from build123d import *

# Parameters (mm, degrees)
SALIENTE_EXTRUIR1_DEPTH = 10
CROQUIS2_R              = 2
CORTAR_EXTRUIR1_DEPTH   = 10
CROQUIS3_R              = 2
CORTAR_EXTRUIR2_DEPTH   = 10


with BuildPart() as part:
    # Croquis1 → Saliente-Extruir1 (new body)
    with BuildSketch(Plane(origin=(0, 0, 0), x_dir=(0, 0, -1), z_dir=(1, 0, 0))):
        Polygon((0, 0), (37.42423058, 37.42423058), (50, 0), align=None)
    extrude(amount=SALIENTE_EXTRUIR1_DEPTH)

    # Croquis2 → Cortar-Extruir1 (cut)
    with BuildSketch(Plane.XZ):
        with Locations(Location((5, -34.477712546, 0), (0, 0, 270))):
            Circle(CROQUIS2_R)
    extrude(amount=-CORTAR_EXTRUIR1_DEPTH, mode=Mode.SUBTRACT)

    # Croquis3 → Cortar-Extruir2 (cut)
    with BuildSketch(Plane(origin=(0, 0, 0), x_dir=(1, 0, 0), z_dir=(0, 0.7071067811865512, 0.7071067811865439))):
        with Locations(Location((5, 42.766502378, 0), (0, 0, 270))):
            Circle(CROQUIS3_R)
    extrude(amount=-CORTAR_EXTRUIR2_DEPTH, mode=Mode.SUBTRACT)


solid = part.part
The listing builds one solid part. Answer for the finished solid, in the listing's coordinates (mm). A direction names the side the tool comes from. Give positions to 0.01 mm unless a question says otherwise; leave off trailing zeros. Loops run counter-clockwise (first coordinate to the right, second up) from the corner with the lowest first, then second, coordinate; pieces in that order, holes last.
Item 1: Each of these flat-tipped pins is pushed along its axis until it touches: pin 1 Ø6 at (x, y) = (6.5, 12.5) entering from +Z; pin 2 Ø2 at (x, y) = (6.5, 11.5) entering from -Z; pin 3 Ø3 at (x, z) = (5, -34.48) entering from +Y. Where does it stop, or does it pass through?
Derived:
pin 1: stops at z = -9.5
pin 2: stops at z = -46.47
pin 3: stops at y = 35.98
Item 2: A cutting plane is placed at D-D (x = 1). Give the vertices of the cut face in (y, z).
Derived:
outline: (0, -50) - (37.42, -37.42) - (0, 0) - close
Item 3: A tool of negligible diameter and unlimited length cuts with its end or side. For faces 1 (the flat face through (0, 11, -31)), 2 (the flat face through (5.03, 23.19, -37.33)), 3 (the flat face through (5, 10, -34)), from which of +Z, -Z, +X, -X, +Y, -Y can it reach the whole face along a straight path? Write none if from no direction.
Derived:
face 1: +Z, -Z, -X, +Y, -Y
face 2: none
face 3: -Y
Item 4: Find the intervals of material crossed by line 1 along Z through (x, y) = (3.5, 28); line 2 along Y through (x, z) = (8.5, -10); line 3 along Z through (x, y) = (3, 16.5), in increasing order.
Derived:
line 1: z = -40.59 to -34.35, -30.61 to -28
line 2: y = 0 to 10
line 3: z = -44.46 to -16.5
Item 5: A cutting plane is placed at B-B (z = -21). Give the vertices of the cut face in (x, y), then the cut area to 3 significant figures.
Derived:
outline: (0, 0) - (10, 0) - (10, 21) - (0, 21) - close
area: 210 mm2
Item 6: Determine the mould class of faces 4 (the cylindrical face through (5.601, 4.93, -36.385)), 5 (the flat face through (5, 0, -25)), 6 (the cylindrical face through (6.35, 27.8, -34.77)) for opening direction Y: +Y half, -Y half, draft (parallel to the pull), parting line (faces both ways), or undercut.
Derived:
face 4: draft
face 5: -Y half
face 6: undercut
Item 7: A cutting plane is placed at A-A (x = 5). Give the vertices of the cut face in (y, z).
Derived:
outline: (0, -50) - (37.42, -37.42) - (31.65, -31.65) - (24.58, -38.73) - (21.76, -35.9) - (28.83, -28.83) - (0, 0) - (0, -32.48) - (10, -32.48) - (10, -36.48) - (0, -36.48) - close
Item 8: A cutting plane is placed at C-C (y = 14.5). Give the vertices of the cut face in (x, z), then the cut area to 3 significant figures.
Derived:
outline: (0, -45.13) - (10, -45.13) - (10, -14.5) - (0, -14.5) - close
area: 306 mm2
